Can you work these out from the model? Positions are in its coordinate system, mm. A direction names the side the tool comes from. Give positions to 0.01 mm unless a question says otherwise; leave off trailing zeros. Loops run counter-clockwise (first coordinate to the right, second up) from the corner with the lowest first, then second, coordinate; pieces in that order, holes last. Notation, with made-up numbers: (-20.75, -36.5) - (-9.75, -36.5) arc R18 cw to (-9.75, -1.5) - close; hole circle Ø9 at (-25.5, -31). An arc over 180 degrees is marked (long way). Use a Markdown table: item, result. Add a question column.
```python
from build123d import *

# Parameters (mm, degrees)
BOSS_EXTRUDE1_DEPTH  = 105
M4_CLEARANCE_HOLE2_D = 4.5


with BuildPart() as part:
    # Sketch1 → Boss-Extrude1 (new body)
    with BuildSketch(Plane.XY):
        Polygon((-6.604, 0), (6.604, 0), (6.604, -12.7), (5.0165, -12.7), (5.0165, -1.5875), (-5.0165, -1.5875), (-5.0165, -12.7), (-6.604, -12.7), align=None)
    extrude(amount=-BOSS_EXTRUDE1_DEPTH)

    # M4 Clearance Hole2 (through all)
    with Locations(Plane(origin=(0, 0, 0), x_dir=(1, 0, 0), z_dir=(0, 1, 0))):
        with Locations((0, 56.807786), (0, 30), (0, 76.807786)):
            Hole(M4_CLEARANCE_HOLE2_D / 2)


solid = part.part
```
1. Suppose I cut it at B-B (y = -10.25). List the corners of the cut face in (x, z) for me, and give its area (3 significant figures).
2. If we mould it in two halves opening along Z, with no side actions, what happens to faces 3 (the face through (1, -1, 0)), 4 (the face through (0, -1.588, -52)), 5 (the face through (-1.038, -0.805, -54.812)), 6 (the face through (0.488, -0.805, -27.804))? For each: released by +Z, released by -Z, zero draft, split by the parting line, or undercut.
3. Please list where these lines run through material, in increasing order: line 1 along Z through (x, y) = (0, -0.4); line 2 along X through (y, z) = (-11, -13.5); line 3 along X through (y, z) = (-0.7, -30). Write a range as [from, to].
4. Suppose I cut it at D-D (z = -71). List the corners of the cut face in (x, y) for me.
5. Suppose I cut it at C-C (z = -30). List the corners of the cut face in (x, y) for me.
6. Will these pins go through, and if not, where does the flat tip stop? P1, Ø6, axis at x = 1.5, y = -1.5, coming from the +Z side; P2, Ø7, axis at x = 0, z = -30, coming from the -Y side.
7. Suppose I cut it at A-A (x = 0). List the corners of the cut face in (y, z) for me.
8. On a 3-axis mill with a long thin cutter (end or side, diameter ignored), from which of +Z, -Z, +X, -X, +Y, -Y can I reach the whole of each face in a straight line? I mean faces 1 (the face through (-5.016, -7, -52)), 2 (the face through (6.604, -6, -52)). Say none if no direction works.
Results below:
| question | item | result |
|---|---|---|
| 1 | outline | (-6.6, -105) - (-5.02, -105) - (-5.02, 0) - (-6.6, 0) - close; (5.02, -105) - (6.6, -105) - (6.6, 0) - (5.02, 0) - close |
| 1 | area | 333 mm² |
| 2 | face 3 | released by +Z |
| 2 | face 4 | zero draft |
| 2 | face 5 | undercut |
| 2 | face 6 | undercut |
| 3 | line 1 | [-105, -79.06], [-74.56, -59.06], [-54.56, -32.25], [-27.75, 0] |
| 3 | line 2 | [-6.6, -5.02], [5.02, 6.6] |
| 3 | line 3 | [-6.6, -2.25], [2.25, 6.6] |
| 4 | outline | (-6.6, -12.7) - (-5.02, -12.7) - (-5.02, -1.59) - (5.02, -1.59) - (5.02, -12.7) - (6.6, -12.7) - (6.6, 0) - (-6.6, 0) - close |
| 5 | outline | (-6.6, -12.7) - (-5.02, -12.7) - (-5.02, -1.59) - (-2.25, -1.59) - (-2.25, 0) - (-6.6, 0) - close; (2.25, -1.59) - (5.02, -1.59) - (5.02, -12.7) - (6.6, -12.7) - (6.6, 0) - (2.25, 0) - close |
| 6 | P1 | z = 0 |
| 6 | P2 | y = -1.59 |
| 7 | outline | (-1.59, -105) - (0, -105) - (0, -79.06) - (-1.59, -79.06) - close; (-1.59, -74.56) - (0, -74.56) - (0, -59.06) - (-1.59, -59.06) - close; (-1.59, -54.56) - (0, -54.56) - (0, -32.25) - (-1.59, -32.25) - close; (-1.59, -27.75) - (0, -27.75) - (0, 0) - (-1.59, 0) - close |
| 8 | face 1 | +Z, -Z, -Y |
| 8 | face 2 | +Z, -Z, +X, +Y, -Y |
